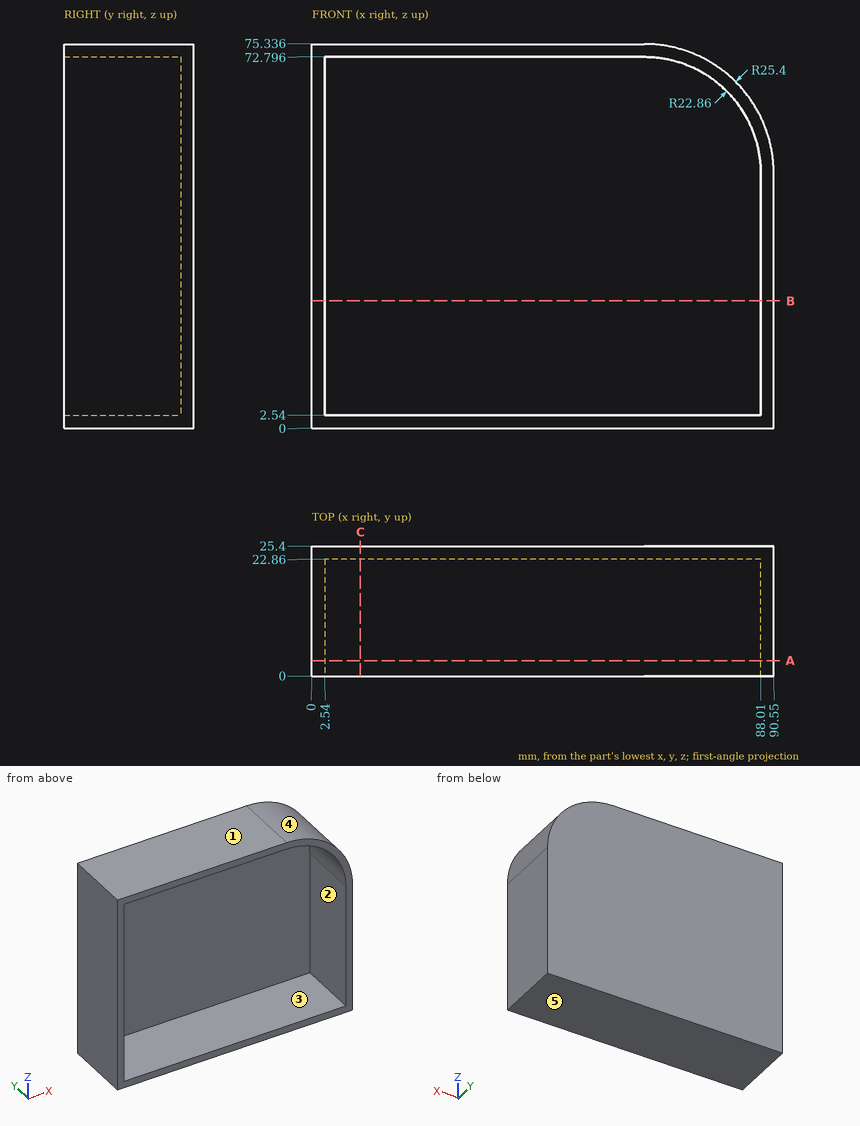
Can you work these out from the drawing? Everything is in mm from the part's minimum corner. A direction names the side the tool comes from. Round coordinates to 2 decimals unless told otherwise and drop trailing zeros. Loops run counter-clockwise (first coordinate to the right, second up) from the corner with the lowest first, then second, coordinate; pieces in that order, holes last. Notation, with made-up numbers: (-18, -18.75) - (31, -18.75) arc R12 ccw to (31, -6.75) - close; hole circle Ø1 at (44, 44.5). An arc over 180 degrees is marked (long way). One line per question, with ' | ' between items. Start each with the question number.
Q1. Please list where these lines run through material, in increasing order: line 1 (Z direction, x = 54, y = 1); line 2 (X direction, y = 7.75, z = 48); line 3 (Y direction, x = 86, z = 3). Write a range as [from, to].
Q2. For the marked faces 1 and 2, which set-ups out of +Z, -Z, +X, -X, +Y, -Y let a thin tool reach every point of the face, with its end or its side?
Q3. I want a section at C-C (x = 9.5). Write out the boundary of the cut face in (y, z).
Q4. I want a section at B-B (z = 25). Write out the boundary of the cut face in (x, y), then the cut area to 3 significant figures.
Q5. I want a section at A-A (y = 3). Write out the boundary of the cut face in (x, z).
Q6. We'd pull the mould along X, two halves only. Please class the marked faces 3, 4 and 5: +X half, -X half, draft (parallel to the pull), parting line (faces both ways), or undercut.
Q7. Will these pins go through, and if not, where does the flat tip stop? pin 1 (8 mm diameter, centred on y = 5, z = 64, fed in from -X); pin 2 (3 mm diameter, centred on x = 36, z = 61.5, fed in from -Y).
Response values:
1) line 1: z = [0, 2.54], [72.8, 75.34] | line 2: x = [0, 2.54], [88.01, 90.55] | line 3: y = [22.86, 25.4]
2) face 1: +Z, +X, -X, +Y, -Y | face 2: -Y
3) outline: (0, 0) - (25.4, 0) - (25.4, 75.34) - (0, 75.34) - (0, 72.8) - (22.86, 72.8) - (22.86, 2.54) - (0, 2.54) - close
4) outline: (0, 0) - (2.54, 0) - (2.54, 22.86) - (88.01, 22.86) - (88.01, 0) - (90.55, 0) - (90.55, 25.4) - (0, 25.4) - close | area: 346 mm²
5) outline: (0, 0) - (90.55, 0) - (90.55, 49.94) arc R25.4 ccw to (65.15, 75.34) - (0, 75.34) - close; hole (2.54, 2.54) - (88.01, 2.54) - (88.01, 49.94) arc R22.86 ccw to (65.15, 72.8) - (2.54, 72.8) - close
6) face 3: undercut | face 4: +X half | face 5: draft
7) pin 1: stops at x = 0 | pin 2: stops at y = 22.86
